Could you check a few things on this model? Use its own coordinates, in mm. Face numbers are marked on the shaded views. Give positions to 0.01 mm unless a question says otherwise; leave off trailing zeros. Write each question's results on one line, items separated by ' | '. Start each with the question number.
from build123d import *

# Parameters (mm, degrees)
PAD005_DEPTH    = 10
SKETCH015_R     = 3.125
SKETCH015_R_2   = 1.25
PAD006_DEPTH    = 110
SKETCH016_W     = 88
SKETCH016_H     = 11
POCKET006_DEPTH = 10.001
SKETCH017_W     = 20
SKETCH017_H     = 10
PAD007_DEPTH    = 5
POCKET007_DEPTH = 85.509727
SKETCH019_R     = 5.5
POCKET008_DEPTH = 75
FILLET_R        = 1.75


with BuildPart() as part:
    # Sketch014 → Pad005 (new body)
    with BuildSketch(Plane.XY):
        with BuildLine():
            Line((55.320782, -4.5), (50.377184, -4.5))
            add(Edge.make_bspline(
                [(50.377184, -4.5), (53.986589, 28.285571), (45.809605, 54.91681), (30.437237, 68.919253), (14.05506, 72.999995), (2.4e-05, 73), (-14.058167, 73.000005), (-30.444405, 68.917468), (-45.797003, 54.963624), (-53.960317, 28.337681), (-50.332268, -4.5)],
                knots=[0.459879, 0.459879, 0.459879, 0.459879, 0.459879, 0.459879, 1, 1, 1, 1, 1, 1.540216, 1.540216, 1.540216, 1.540216, 1.540216, 1.540216], degree=5, weights=[1.511377, 1.459145, 1.581492, 1.878748, 2.351855, 3, 2.351741, 1.878582, 1.580192, 1.456955, 1.509005]))
            Line((-50.332268, -4.5), (-55.312029, -4.5))
            add(Edge.make_bspline(
                [(55.320782, -4.5), (59.190875, 30.481044), (50.18289, 58.805264), (33.344109, 73.658439), (15.399277, 77.999995), (2.5e-05, 78), (-15.399851, 78.000005), (-33.345502, 73.658102), (-50.180453, 58.814098), (-59.185767, 30.490915), (-55.312029, -4.5)],
                knots=[0.460805, 0.460805, 0.460805, 0.460805, 0.460805, 0.460805, 1, 1, 1, 1, 1, 1.539212, 1.539212, 1.539212, 1.539212, 1.539212, 1.539212], degree=5, weights=[1.509472, 1.458717, 1.582334, 1.880371, 2.352966, 3, 2.352945, 1.88034, 1.582103, 1.458328, 1.50905]))
        make_face()
    extrude(amount=PAD005_DEPTH)

    # Sketch015 (on DatumPlane) → Pad006 (join)
    with BuildSketch(Plane(origin=(55.001235, 46.003648, 5), x_dir=(0, 0, -1), z_dir=(1, -4.6e-05, 0))):
        with Locations((0, -46.2)):
            Circle(SKETCH015_R)
        with Locations((1.8, -44.4)):
            Circle(SKETCH015_R_2)
    extrude(amount=-PAD006_DEPTH)

    # Sketch016 (on Face5 of Pad006) → Pocket006 (cut, through all)
    with BuildSketch(Plane.XY.offset(10)):
        Rectangle(SKETCH016_W, SKETCH016_H)
    extrude(amount=-POCKET006_DEPTH, mode=Mode.SUBTRACT)

    # Sketch017 (on DatumPlane) → Pad007 (join)
    with BuildSketch(Plane(origin=(0.002608, 76.006164, 5), x_dir=(1, -4.6e-05, 0), z_dir=(4.6e-05, 1, 0))):
        Rectangle(SKETCH017_W, SKETCH017_H)
    extrude(amount=PAD007_DEPTH)

    # Sketch018 (on Face14 of Pad007) → Pocket007 (cut, through all)
    with BuildSketch(Plane(origin=(0.003707, 81.006164, 10), x_dir=(1, -4.6e-05, 0), z_dir=(4.6e-05, 1, 0))):
        with BuildLine():
            ThreePointArc((-3.225332, 4.600332), (-3.320764, 2.011977), (-0.781754, 1.5))
            Line((-0.781754, 1.5), (0.781754, 1.5))
            ThreePointArc((0.781754, 1.5), (3.320764, 2.011977), (3.225332, 4.600332))
            ThreePointArc((3.225332, 4.600332), (0, 8.25), (-3.225332, 4.600332))
        make_face()
    extrude(amount=-POCKET007_DEPTH, mode=Mode.SUBTRACT)

    # Sketch019 → Pocket008 (cut)
    with BuildSketch(Plane.XZ):
        with Locations((0, 5)):
            Circle(SKETCH019_R)
    extrude(amount=-POCKET008_DEPTH, mode=Mode.SUBTRACT)

    # Fillet
    fillet_edges = [part.edges().sort_by_distance(p)[0] for p in [
        (10.002837, 81.005707, 4.999997),
        (10.002661, 77.167792, 4.999997),
        (-9.997339, 77.168929, 5.000003),
        (-9.997163, 81.006622, 5.000003),
    ]]
    fillet(fillet_edges, radius=FILLET_R)


with BuildPart() as part_1:
    # Body004 placement: moved
    add(part.part.moved(Location((0, 0, 2.5))))


solid = part_1.part
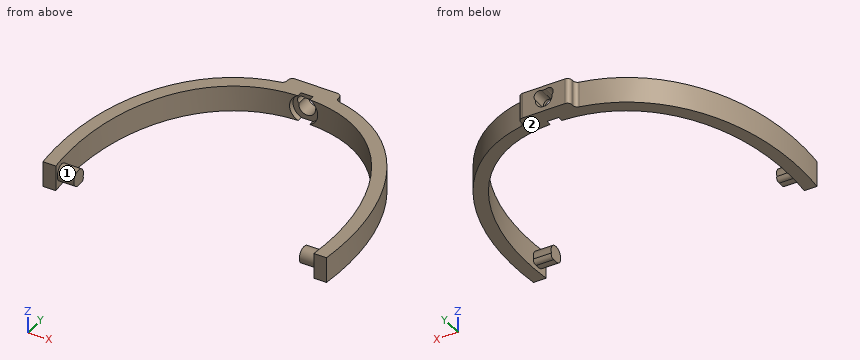
1) Please list where these lines run through material, in increasing order: line 1 (X direction, y = 78.5, z = 7.5); line 2 (X direction, y = 6, z = 10.75); line 3 (Y direction, x = -3.5, z = 7). Write a range as from..to.
2) Thinking about a two-plate mould opening in Y: for the marked faces 1 and 2, which applies, pulls with the +Y half, pulls with the -Y half, needs draft (parallel to the pull), parting line crosses it, or undercut?
3) I'm going to push a flat-ended pin straight in: P1, Ø0.5, axis at y = 79, z = 7.5, coming from the -X side. Where does the tip first touch, or does it pass through?
Calculated:
1) line 1: x = -10..-3.25, 3.25..10.01 | line 2: x = -55.98..-50.98, 51.02..55.99 | line 3: y = 75..81.01
2) face 1: undercut | face 2: needs draft
3) P1: stops at x = -10
